Verification items for this drawing (mm, ordinates from the low corner). A direction names the side the tool comes from. Coordinates: 2 decimals unless noted, no trailing zeros. Write each loop counter-clockwise with the first axis right and the second up, starting at its lowest first coordinate (ties: lowest second). Pieces come first, ordered by that corner, then holes. Notation, with made-up numbers: M -38,76 L -24,76 A16 ccw -24,82 Z; hole C 27.25,33 d11. An arc over 180 degrees is marked long. Write each question's results on one line, items separated by ' | '.
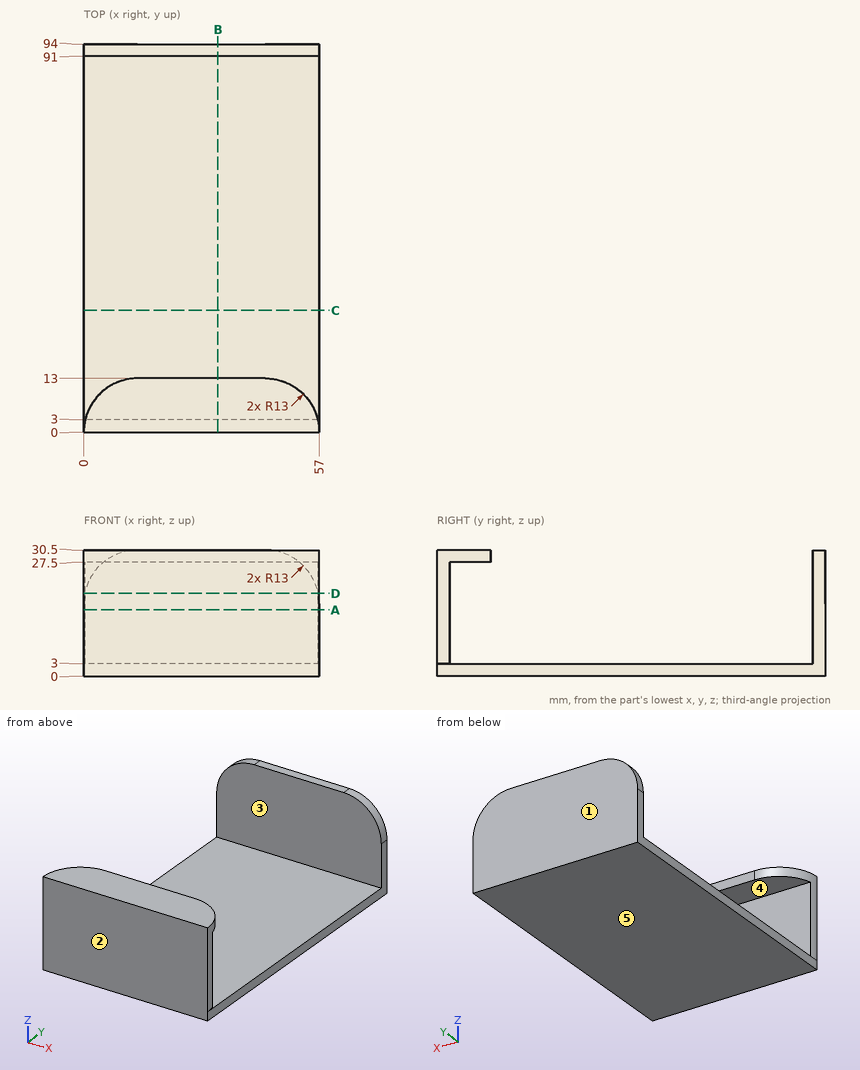
Q1. Sectioned sample at C-C on y = 29.5. Record the cut outline in (x, z), and give its area (3 significant figures).
Geometry check:
outline: M 0,0 L 57,0 L 57,3 L 0,3 Z | area: 171 mm2
Q2. Mould release check, pull along Y, two halves, no side actions. Record for the marked faces 1, 2 and 3: pulls with the +Y half, pulls with the -Y half, needs draft (parallel to the pull), parting line crosses it, or undercut.
Geometry check:
face 1: pulls with the +Y half | face 2: pulls with the -Y half | face 3: undercut
Q3. Sectioned sample at B-B on x = 32.5. Record the cut outline in (y, z).
Geometry check:
outline: M 0,0 L 94,0 L 94,30.5 L 91,30.5 L 91,3 L 3,3 L 3,27.5 L 13,27.5 L 13,30.5 L 0,30.5 Z
Q4. Sectioned sample at D-D on z = 20. Record the cut outline in (x, y), and give its area (3 significant figures).
Geometry check:
outline: M 0,0 L 57,0 A13 ccw 56.65,3 L 0.35,3 A13 ccw Z; M 0.24,91 L 56.76,91 L 56.76,94 L 0.24,94 Z | area: 340 mm2
Q5. Access from +Z, -Z, +X, -X, +Y, -Y to the whole of each face (thin tool, end or side, straight path). Record for the marked faces 4 and 5.
Geometry check:
face 4: +X, -X | face 5: -Z, +X, -X, +Y, -Y
Q6. Depth check by flat-ended pin: P1, Ø8, axis at x = 17.5, y = 38.5, coming from the +Z side; P2, Ø3, axis at x = 9.5, z = 7.5, coming from the -Y side. Enter the tip coordinate at first touch or a pass-through.
Geometry check:
P1: stops at z = 3 | P2: stops at y = 0
Q7. Scan lines: probe 1 along Y at (x, z) = (12.5, 19.5); probe 2 along Z at (x, y) = (24, 77); probe 3 along Y at (x, z) = (30.5, 29). Record each from-to range of solid material in increasing order.
Geometry check:
probe 1: y = 0 to 3, 91 to 94 | probe 2: z = 0 to 3 | probe 3: y = 0 to 13, 91 to 94
Q8. Sectioned sample at A-A on z = 16. Record the cut outline in (x, y), and give its area (3 significant figures).
Geometry check:
outline: M 0,0 L 57,0 A13 ccw 56.65,3 L 0.35,3 A13 ccw Z; M 0,91 L 57,91 L 57,94 L 0,94 Z | area: 341 mm2
